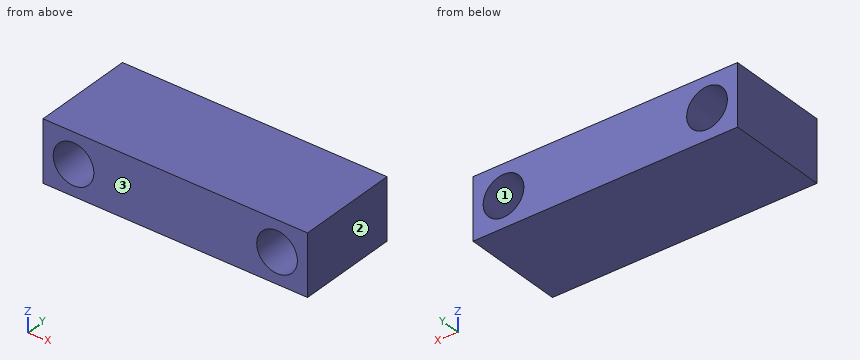
Autodesk Inventor part; units mm, degrees
ref_plane "YZ Plane" through (0, 0, 0) normal (1, 0, 0) x (0, 1, 0)
ref_plane "XZ Plane" through (0, 0, 0) normal (0, 1, 0) x (-1, 0, 0)
ref_plane "XY Plane" through (0, 0, 0) normal (0, 0, 1) x (1, 0, 0)
sketch "Sketch1" plane through (0, 0, 0) normal (0, 1, 0) x (-1, 0, 0)
  line L0 (-6.5, -1.5) -> (6.5, -1.5)
  line L1 (6.5, 3.5) -> (6.5, 3.5)
  line L2 (6.5, 1.5) -> (-6.5, 1.5)
  line L3 (-6.5, 3.5) -> (-6.5, 3.5)
  line L4 (-6.5, -1.5) -> (6.5, 1.5) construction
  line L5 (6.5, -1.5) -> (-6.5, 1.5) construction
  circle A0 centre (5, 0) radius 1
  line L6 (-6.5, 1.5) -> (-6.5, -1.5)
  line L7 (6.5, 1.5) -> (6.5, -1.5)
  line L8 (-6.5, 1.5) -> (-7.5, 1.5)
  circle A1 centre (-5, 0) radius 1
  point P0 (0, 0)
  dimension "d0" = 3
  dimension "d1" = 13
  dimension "d3" = 2
  dimension "d6" = 1.5
  dimension "d8" = 1.5
  dimension "d21" = 2
  dimension "d22" = 1.5
  dimension "d23" = 1.5
extrude "Extrusion1" add sketch "Sketch1" along normal blind 5
properties part number "link"
Check sheet for the modelled part. Datum: model origin and axes. Units: mm. Face numbers are marked on the shaded views. Round coordinates to 2 decimals unless told otherwise and drop trailing zeros. Order: outer loops, then holes, each group sorted by start corner. A loop starts at its lowest first (then second) coordinate and runs counter-clockwise, first axis right, second up.
Q1. Cross-section at B-B, the plane x = 5. Enter the section's corners in (y, z), plus the area to 3 significant figures.
Filled sheet:
outline: (0, -1.5) - (5, -1.5) - (5, -1) - (0, -1) - close; (0, 1) - (5, 1) - (5, 1.5) - (0, 1.5) - close
area: 5.00 mm2
Q2. Depth check by flat-ended pin: P1, Ø1.2, axis at x = -5, z = 0, coming from the +Y side. Enter the tip coordinate at first touch or a pass-through.
Filled sheet:
P1: passes through
Q3. Cross-section at C-C, the plane y = 1.8. Enter the section's corners in (x, z), plus the area to 3 significant figures.
Filled sheet:
outline: (-6.5, -1.5) - (6.5, -1.5) - (6.5, 1.5) - (-6.5, 1.5) - close; hole circle Ø2 at (-5, 0); hole circle Ø2 at (5, 0)
area: 32.7 mm2
Q4. Scan lines: L1, parallel to X at y = 0.75, z = 0.75; L2, parallel to X at y = 3.5, z = 0.2; L3, parallel to Z at x = -5, y = 3.85. Record each from-to range of solid material in increasing order.
Filled sheet:
L1: x = -6.5 to -5.66, -4.34 to 4.34, 5.66 to 6.5
L2: x = -6.5 to -5.98, -4.02 to 4.02, 5.98 to 6.5
L3: z = -1.5 to -1, 1 to 1.5
Q5. Cross-section at D-D, the plane z = 0. Enter the section's corners in (x, y).
Filled sheet:
outline: (-6.5, 0) - (-6, 0) - (-6, 5) - (-6.5, 5) - close; (-4, 0) - (4, 0) - (4, 5) - (-4, 5) - close; (6, 0) - (6.5, 0) - (6.5, 5) - (6, 5) - close
Q6. Draft check along X on the marked faces 1, 2 and 3. Enter one of: pulls with the +X half, pulls with the -X half, needs draft (parallel to the pull), parting line crosses it, or undercut.
Filled sheet:
face 1: undercut
face 2: pulls with the +X half
face 3: needs draft
Q7. Cross-section at A-A, the plane z = -0.6. Enter the section's corners in (x, y).
Filled sheet:
outline: (-6.5, 0) - (-5.8, 0) - (-5.8, 5) - (-6.5, 5) - close; (-4.2, 0) - (4.2, 0) - (4.2, 5) - (-4.2, 5) - close; (5.8, 0) - (6.5, 0) - (6.5, 5) - (5.8, 5) - close
